CAD build for the part. Positions are in the model's coordinates, mm. A direction names the side the tool comes from. Coordinates: 2 decimals unless noted, no trailing zeros. Order: outer loops, then holes, each group sorted by start corner. A loop starts at its lowest first (then second) coordinate and runs counter-clockwise, first axis right, second up. Notation, with made-up numbers: (31.5, 83) - (70.5, 83) arc R32 ccw to (70.5, 117) - close; hole circle Ø1 at (-9, 24.25). An arc over 180 degrees is marked (long way). Return JSON: item names as keys, results as strings.
from build123d import *

# Parameters (mm, degrees)
SKETCH_1_R          = 7.5
EXTRUDE_1_DEPTH     = 0.8
SKETCH_2_R          = 5.5
EXTRUDE_2_DEPTH     = 9.3
SKETCH_3_R          = 7.6
EXTRUDE_3_DEPTH     = 7.4
SKETCH_4_R          = 2.5
CUT_EXTRUDE_1_DEPTH = 21.537039709


with BuildPart() as part:
    # Эскиз1 → Бобышка-Вытянуть1 (new body)
    with BuildSketch(Plane.XY):
        Circle(SKETCH_1_R)
    extrude(amount=EXTRUDE_1_DEPTH)

    # Эскиз2 → Бобышка-Вытянуть2 (add)
    with BuildSketch(Plane.XY.offset(0.8)):
        Circle(SKETCH_2_R)
    extrude(amount=EXTRUDE_2_DEPTH)

    # Эскиз3 → Бобышка-Вытянуть3 (add)
    with BuildSketch(Plane.XY.offset(10.1)):
        Circle(SKETCH_3_R)
    extrude(amount=EXTRUDE_3_DEPTH)

    # Эскиз4 → Вырез-Вытянуть1 (cut, through all)
    with BuildSketch(Plane.XY.offset(17.5)):
        Circle(SKETCH_4_R)
    extrude(amount=-CUT_EXTRUDE_1_DEPTH, mode=Mode.SUBTRACT)


solid = part.part
Item 1: Drop flat-ended pins along their axis: P1, Ø2, axis at y = -5.5, z = 14.5, coming from the +X side; P2, Ø3, axis at x = -5.5, z = 15, coming from the -Y side; P3, Ø4, axis at x = 3.5, z = 15, coming from the -Y side. Give the stop position or say it passes through.
Findings below:
{"P1": "stops at x = 6.12", "P2": "stops at y = -6.46", "P3": "stops at y = -7.45"}
Item 2: Mould opens along Z. For faces 3 (the flat face through (-2, 2, 17.5)), 4 (the flat face through (-4, 4, 0.8)), 5 (the cylindrical face through (-7.493, 0.33, 0.394)) say: released by +Z, released by -Z, zero draft, split by the parting line, or undercut.
Findings below:
{"face 3": "released by +Z", "face 4": "undercut", "face 5": "zero draft"}
Item 3: Band-saw the part on D-D, the plane x = 2.75. List the corners of the cut face in (y, z).
Findings below:
{"outline": "(-7.09, 10.1) - (-4.76, 10.1) - (-4.76, 0.8) - (-6.98, 0.8) - (-6.98, 0) - (6.98, 0) - (6.98, 0.8) - (4.76, 0.8) - (4.76, 10.1) - (7.09, 10.1) - (7.09, 17.5) - (-7.09, 17.5) - close"}
Item 4: Which spindle directions (+Z, -Z, +X, -X, +Y, -Y) get a long thin tool onto all of the face, cutting with end or side? Do faces 1 (the flat face through (-2, 2, 0)), 2 (the flat face through (4, 4, 10.1)). Say none if no direction does.
Findings below:
{"face 1": "-Z, +X, -X, +Y, -Y", "face 2": "none"}
Item 5: Band-saw the part on C-C, the plane z = 12. List the corners of the cut face in (x, y).
Findings below:
{"outline": "circle Ø15.2 at (0, 0); hole circle Ø5 at (0, 0)"}
Item 6: Band-saw the part on A-A, the plane y = 0. List the corners of the cut face in (x, z).
Findings below:
{"outline": "(-7.6, 10.1) - (-5.5, 10.1) - (-5.5, 0.8) - (-7.5, 0.8) - (-7.5, 0) - (-2.5, 0) - (-2.5, 17.5) - (-7.6, 17.5) - close; (2.5, 0) - (7.5, 0) - (7.5, 0.8) - (5.5, 0.8) - (5.5, 10.1) - (7.6, 10.1) - (7.6, 17.5) - (2.5, 17.5) - close"}
Item 7: Wall check: L1, parallel to Y at x = 0, z = 13.75; L2, parallel to Z at x = -5, y = -3.5; L3, parallel to Y at x = 0, z = 7.75. Give the ranges that are in metal, low to high. Write a range as [from, to].
Findings below:
{"L1": "y = [-7.6, -2.5], [2.5, 7.6]", "L2": "z = [0, 0.8], [10.1, 17.5]", "L3": "y = [-5.5, -2.5], [2.5, 5.5]"}
